Input: part model. Units: mm. Frame: model coordinates. Round coordinates to 2 decimals unless told otherwise and drop trailing zeros. Use one line per item in the form item = value. Start each with the question number.
```python
from build123d import *

# Parameters (mm, degrees)
SKETCH1_W           = 100
SKETCH1_H           = 75
BOSS_EXTRUDE1_DEPTH = 3
FILLET1_R           = 10
SKETCH2_R           = 1
CUT_EXTRUDE1_DEPTH  = 4


with BuildPart() as part:
    # Sketch1 → Boss-Extrude1 (new body)
    with BuildSketch(Plane(origin=(0, 0, 0), x_dir=(1, 0, 0), z_dir=(0, 1, 0))):
        Rectangle(SKETCH1_W, SKETCH1_H)
    extrude(amount=BOSS_EXTRUDE1_DEPTH)

    # Fillet1
    fillet1_edges = [part.edges().sort_by_distance(p)[0] for p in [
        (50, 1.5, 37.5),
        (-50, 1.5, 37.5),
    ]]
    fillet(fillet1_edges, radius=FILLET1_R)

    # Sketch2 → Cut-Extrude1 (cut, through all)
    with BuildSketch(Plane(origin=(0, 3, 0), x_dir=(1, 0, 0), z_dir=(0, 1, 0))):
        with Locations((38.351170888, -31)):
            Circle(SKETCH2_R)
    cut_extrude1 = extrude(amount=-CUT_EXTRUDE1_DEPTH, mode=Mode.SUBTRACT)

    # Mirror1: Cut-Extrude1 across plane
    add(cut_extrude1.mirror(Plane.XY), mode=Mode.SUBTRACT)


solid = part.part
```
Item 1: Ray query, line 1 (X direction, y = 2.15, z = -31); line 2 (X direction, y = 1.6, z = 31); line 3 (X direction, y = 1, z = 34). Return the intervals inside material, ascending. Write a range as from..to.
Item 2: Draft query along Z for faces 1 (the face through (39.305, 1.521, 30.7)), 2 (the face through (-1, 0, -1)), 3 (the face through (-1, 1, -37.5)), 4 (the face through (-47.15, 1.52, 34.49)). Return one class per face: +Z half, -Z half, draft (parallel to the pull), parting line (faces both ways), or undercut.
Item 3: First-contact query: pin 1 (1.2 mm diameter, centred on x = 38.35, z = 31, fed in from +Y). Flat tip, straight axial feed; report the tip coordinate or a pass-through.
Final values:
q1.line_1 = -50..37.35, 39.35..50
q1.line_2 = -49.37..37.35, 39.35..49.37
q1.line_3 = -47.6..47.6
q2.face_1 = undercut
q2.face_2 = draft
q2.face_3 = -Z half
q2.face_4 = +Z half
q3.pin_1 = through
